Could you check a few things on this model? Use its own coordinates, in mm. A direction names the side the tool comes from. Coordinates: 2 decimals unless noted, no trailing zeros. Loops run counter-clockwise (first coordinate to the right, second up) from the corner with the lowest first, then second, coordinate; pieces in that order, holes last. Notation, with made-up numbers: M 70,16 L 102,16 A17 cw 102,23 Z; hole C -35.5,-8.5 d6. An arc over 180 degrees is marked long. Write each question's results on one line, items separated by ' | '.
Autodesk Inventor part; units mm, degrees
ref_plane "YZ Plane" through (0, 0, 0) normal (1, 0, 0) x (0, 1, 0)
ref_plane "XZ Plane" through (0, 0, 0) normal (0, 1, 0) x (-1, 0, 0)
ref_plane "XY Plane" through (0, 0, 0) normal (0, 0, 1) x (1, 0, 0)
sketch "Szkic1" plane through (0, 0, 0) normal (0, 1, 0) x (-1, 0, 0)
  line L0 (-12.7, 166.37) -> (-12.7, -10.16)
  line L1 (-10.16, -12.7) -> (12.7, -12.7)
  line L2 (15.24, -10.16) -> (15.24, -2.54)
  line L3 (12.7, 0) -> (2.54, 0)
  line L4 (0, 2.54) -> (0, 166.37)
  line L5 (-2.54, 168.91) -> (-10.16, 168.91)
  line L6 (-6.35, 168.91) -> (-6.35, -12.7) construction
  circle A0 centre (-6.35, 161.29) radius 1.6
  circle A1 centre (-6.35, 125.73) radius 1.6
  circle A2 centre (-6.35, 90.17) radius 1.6
  circle A3 centre (-6.35, 54.61) radius 1.6
  line L7 (15.24, -6.35) -> (-12.7, -6.35) construction
  circle A4 centre (7.62, -6.35) radius 1.6
  circle A5 centre (-6.35, -6.35) radius 1.6
  line L8 (-2.54, 168.91) -> (0, 166.37)
  line L9 (-10.16, 168.91) -> (-12.7, 166.37)
  line L10 (-12.7, -10.16) -> (-10.16, -12.7)
  line L11 (0, 2.54) -> (2.54, 0)
  line L12 (12.7, 0) -> (15.24, -2.54)
  line L13 (12.7, -12.7) -> (15.24, -10.16)
  line L14 (-1, 165.9558) -> (-2.9542, 167.91)
  line L15 (-2.9542, 167.91) -> (-9.7458, 167.91)
  line L16 (-9.7458, 167.91) -> (-11.7, 165.9558)
  line L17 (-11.7, 165.9558) -> (-11.7, -9.7458)
  line L18 (-11.7, -9.7458) -> (-9.7458, -11.7)
  line L19 (-9.7458, -11.7) -> (12.2858, -11.7)
  line L20 (12.2858, -11.7) -> (14.24, -9.7458)
  line L21 (14.24, -9.7458) -> (14.24, -2.9542)
  line L22 (14.24, -2.9542) -> (12.2858, -1)
  line L23 (12.2858, -1) -> (2.1258, -1)
  line L24 (2.1258, -1) -> (-1, 2.1258)
  line L25 (-1, 2.1258) -> (-1, 165.9558)
  point P0 (0, 0)
  point P1 (-12.7, 168.91)
  point P2 (-12.7, -12.7)
  point P3 (15.24, -12.7)
  point P4 (15.24, 0)
  point P5 (0, 0)
  point P6 (0, 168.91)
  dimension "d0" = 12.7
  dimension "d1" = 181.61
  dimension "d2" = 27.94
  dimension "d3" = 3.2
  dimension "d4" = 7.62
  dimension "d7" = 35.56
  dimension "d12" = 3.2
  dimension "d13" = 3.2
  dimension "d14" = 7.62
  dimension "d15" = 2.54
  dimension "d16" = 2.54
  dimension "d17" = 2.54
  dimension "d18" = 2.54
  dimension "d19" = 2.54
  dimension "d20" = 2.54
  dimension "d21" = 2.54
  dimension "d22" = 2.54
  dimension "d23" = 2.54
  dimension "d24" = 2.54
  dimension "d25" = 2.54
  dimension "d26" = 2.54
  dimension "d27" = 1
extrude "Wyciągnięcie proste2" add sketch "Szkic1" along normal blind 3 contours L25 L24 L23 L22 L21 L20 L19 L18 L17 L16 L15 L14
properties part number "bar_+BattPow"
(1) Imagine slicing it at A-A, the plane z = -6.35. List the corners of the cut face in (x, y) for me.
Reported:
outline: M -14.24,0 L -9.22,0 L -9.22,3 L -14.24,3 Z; M -6.02,0 L 4.75,0 L 4.75,3 L -6.02,3 Z; M 7.95,0 L 11.7,0 L 11.7,3 L 7.95,3 Z
(2) Which directions (+Z, -Z, +X, -X, +Y, -Y) give clear straight access to the entire face, cutting with the end or side of a thin tool? Please do faces 1 (the flat face through (-7, 1, -1)), 2 (the cylindrical face through (6.558, 1.479, 124.144)).
Reported:
face 1: +Z, -X, +Y, -Y | face 2: +Y, -Y
(3) Imagine slicing it at C-C, the plane y = 1. List the corners of the cut face in (x, z) for me, and give its area (3 significant figures).
Reported:
outline: M -14.24,-9.75 L -12.29,-11.7 L 9.75,-11.7 L 11.7,-9.75 L 11.7,165.96 L 9.75,167.91 L 2.95,167.91 L 1,165.96 L 1,2.13 L -2.13,-1 L -12.29,-1 L -14.24,-2.95 Z; hole C -7.62,-6.35 d3.2; hole C 6.35,-6.35 d3.2; hole C 6.35,54.61 d3.2; hole C 6.35,90.17 d3.2; hole C 6.35,125.73 d3.2; hole C 6.35,161.29 d3.2 | area: 2,030 mm2
(4) Please list where these lines run through material, in increasing order: probe 1 along Z at (x, y) = (6.35, 0.95); probe 2 along X at (y, z) = (0.8, 161.29); probe 3 along Z at (x, y) = (7.75, 0.9). Write a range as from..to.
Reported:
probe 1: z = -11.7..-7.95, -4.75..53.01, 56.21..88.57, 91.77..124.13, 127.33..159.69, 162.89..167.91 | probe 2: x = 1..4.75, 7.95..11.7 | probe 3: z = -11.7..-7.12, -5.58..53.84, 55.38..89.4, 90.94..124.96, 126.5..160.52, 162.06..167.91
(5) If we mould it in two halves opening along X, with no side actions, what happens to faces 3 (the cylindrical face through (6.7, 1.48, 56.17)), 4 (the flat face through (-14.24, 1, -6)), 5 (the flat face through (5, 3, 79))? For each: released by +X, released by -X, zero draft, split by the parting line, or undercut.
Reported:
face 3: undercut | face 4: released by -X | face 5: zero draft
(6) Imagine slicing it at D-D, the plane z = 161.29. List the corners of the cut face in (x, y) for me, and give its area (3 significant figures).
Reported:
outline: M 1,0 L 4.75,0 L 4.75,3 L 1,3 Z; M 7.95,0 L 11.7,0 L 11.7,3 L 7.95,3 Z | area: 22.5 mm2
(7) Imagine slicing it at B-B, the plane x = -7.62. List the corners of the cut face in (y, z) for me.
Reported:
outline: M 0,-11.7 L 3,-11.7 L 3,-7.95 L 0,-7.95 Z; M 0,-4.75 L 3,-4.75 L 3,-1 L 0,-1 Z
